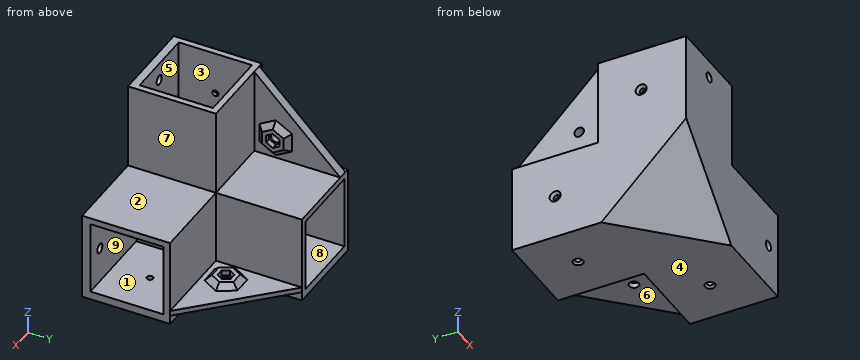
from build123d import *

# Parameters (mm, degrees)
ESQUISSE1_W                                       = 121.6
ESQUISSE1_H                                       = 121.6
BOSS_EXTRU_1_DEPTH                                = 60.8
ESQUISSE2_W                                       = 60.8
ESQUISSE2_H                                       = 60.8
ENL_V_MAT_EXTRU_1_DEPTH                           = 149.928976361
ESQUISSE3_W                                       = 60.8
ESQUISSE3_H                                       = 60.8
ENL_V_MAT_EXTRU_2_DEPTH                           = 106.3086891
ESQUISSE4_W                                       = 60.8
ESQUISSE4_H                                       = 60.8
ENL_V_MAT_EXTRU_3_DEPTH                           = 106.3086891
ESQUISSE5_W                                       = 51.8
ESQUISSE5_H                                       = 51.8
ENL_V_MAT_EXTRU_4_DEPTH                           = 60.8
ESQUISSE6_W                                       = 51.8
ESQUISSE6_H                                       = 51.8
ENL_V_MAT_EXTRU_5_DEPTH                           = 60.8
ESQUISSE7_W                                       = 51.8
ESQUISSE7_H                                       = 51.8
ENL_V_MAT_EXTRU_6_DEPTH                           = 60.8
BOSS_EXTRU_8_DEPTH                                = 1.35
FRAISAGE_POUR_VIS_T_TE_FRAIS_E_BOMB_E_D           = 4.3053
FRAISAGE_POUR_VIS_T_TE_FRAIS_E_BOMB_E_DEPTH       = 20
FRAISAGE_POUR_VIS_T_TE_FRAIS_E_BOMB_E_CSINK_D     = 7.0866
FRAISAGE_POUR_VIS_T_TE_FRAIS_E_BOMB_E_CSINK_ANGLE = 82
FRAISAGE_POUR_VIS_T_TE_FRAIS_E_BOMB_E_TIP         = 1.293442612
FRAISAGE_POUR_VIS_T_TE_FRAIS_E_6_PAN_D            = 4.3053
FRAISAGE_POUR_VIS_T_TE_FRAIS_E_6_PAN_DEPTH        = 20
FRAISAGE_POUR_VIS_T_TE_FRAIS_E_6_PAN_CSINK_D      = 7.7978
FRAISAGE_POUR_VIS_T_TE_FRAIS_E_6_PAN_CSINK_ANGLE  = 82
FRAISAGE_POUR_VIS_T_TE_FRAIS_E_6_PAN_TIP          = 1.293442612
BOSS_EXTRU_3_DEPTH                                = 10
ENL_V_MAT_EXTRU_13_DEPTH                          = 6.35
BOSS_EXTRU_2_DEPTH                                = 10
ENL_V_MAT_EXTRU_12_DEPTH                          = 3.3
D_GAGEMENT_1_42_D                                 = 6.7564
D_GAGEMENT_1_42_DEPTH                             = 20
D_GAGEMENT_1_42_TIP                               = 2.029827343
D_GAGEMENT_1_43_D                                 = 6.7564
D_GAGEMENT_1_43_DEPTH                             = 20
D_GAGEMENT_1_43_TIP                               = 2.029827343
BOSS_EXTRU_5_DEPTH                                = 4
CHANFREIN3_SIZE                                   = 4
BOSS_EXTRU_6_DEPTH                                = 4
CHANFREIN4_SIZE                                   = 4
BOSS_EXTRU_7_DEPTH                                = 1.35
D_GAGEMENT_1_44_D                                 = 6.7564
D_GAGEMENT_1_44_DEPTH                             = 20
D_GAGEMENT_1_44_TIP                               = 2.029827343
CHANFREIN1_START                                  = -108
CHANFREIN1_OUTLINE_W                              = 77
CHANFREIN1_OUTLINE_H                              = 88
CHANFREIN1_DEPTH                                  = 35.773481324


with BuildPart() as part:
    # Esquisse1 → Boss.-Extru.1 (new, symmetric)
    with BuildSketch(Plane.XY):
        Rectangle(ESQUISSE1_W, ESQUISSE1_H)
    extrude(amount=BOSS_EXTRU_1_DEPTH, both=True)

    # Esquisse2 → Enlèv. mat.-Extru.1 (cut, through all)
    with BuildSketch(Plane.XY.offset(60.8)):
        with Locations((30.4, 30.4)):
            Rectangle(ESQUISSE2_W, ESQUISSE2_H)
    extrude(amount=-ENL_V_MAT_EXTRU_1_DEPTH, mode=Mode.SUBTRACT)

    # Esquisse3 → Enlèv. mat.-Extru.2 (cut, through all)
    with BuildSketch(Plane(origin=(0, 0, 0), x_dir=(0, 0, -1), z_dir=(1, 0, 0))):
        with Locations((-30.4, 30.4)):
            Rectangle(ESQUISSE3_W, ESQUISSE3_H)
    extrude(amount=-ENL_V_MAT_EXTRU_2_DEPTH, mode=Mode.SUBTRACT)

    # Esquisse4 → Enlèv. mat.-Extru.3 (cut, through all)
    with BuildSketch(Plane(origin=(0, 0, 0), x_dir=(1, 0, 0), z_dir=(0, 1, 0))):
        with Locations((30.4, -30.4)):
            Rectangle(ESQUISSE4_W, ESQUISSE4_H)
    extrude(amount=-ENL_V_MAT_EXTRU_3_DEPTH, mode=Mode.SUBTRACT)

    # Esquisse5 → Enlèv. mat.-Extru.4 (cut)
    with BuildSketch(Plane.XY.offset(60.8)):
        with Locations((-30.4, -30.4)):
            Rectangle(ESQUISSE5_W, ESQUISSE5_H)
    extrude(amount=-ENL_V_MAT_EXTRU_4_DEPTH, mode=Mode.SUBTRACT)

    # Esquisse6 → Enlèv. mat.-Extru.5 (cut)
    with BuildSketch(Plane(origin=(60.8, 0, 0), x_dir=(0, 0, -1), z_dir=(1, 0, 0))):
        with Locations((30.4, -30.4)):
            Rectangle(ESQUISSE6_W, ESQUISSE6_H)
    extrude(amount=-ENL_V_MAT_EXTRU_5_DEPTH, mode=Mode.SUBTRACT)

    # Esquisse7 → Enlèv. mat.-Extru.6 (cut)
    with BuildSketch(Plane(origin=(0, 60.8, 0), x_dir=(1, 0, 0), z_dir=(0, 1, 0))):
        with Locations((-30.4, 30.4)):
            Rectangle(ESQUISSE7_W, ESQUISSE7_H)
    extrude(amount=-ENL_V_MAT_EXTRU_6_DEPTH, mode=Mode.SUBTRACT)

    # Esquisse40 → Boss.-Extru.8 (add)
    with BuildSketch(Plane(origin=(0, 0, -60.8), x_dir=(-1, 0, 0), z_dir=(0, 0, -1))):
        Polygon((0, 0), (-60.8, 0), (-60.8, -60.8), (60.8, -60.8), (60.8, 60.8), (0, 60.8), align=None)
    extrude(amount=BOSS_EXTRU_8_DEPTH)

    # Fraisage pour vis à tête fraisée bombée #61
    with Locations(Plane(origin=(0, 0, -62.15), x_dir=(-1, 0, 0), z_dir=(0, 0, -1))):
        with Locations((-30.4, -30.4), (30.4, 30.4)):
            CounterSinkHole(FRAISAGE_POUR_VIS_T_TE_FRAIS_E_BOMB_E_D / 2, FRAISAGE_POUR_VIS_T_TE_FRAIS_E_BOMB_E_CSINK_D / 2, depth=FRAISAGE_POUR_VIS_T_TE_FRAIS_E_BOMB_E_DEPTH, counter_sink_angle=FRAISAGE_POUR_VIS_T_TE_FRAIS_E_BOMB_E_CSINK_ANGLE)
            with Locations((0, 0, -(FRAISAGE_POUR_VIS_T_TE_FRAIS_E_BOMB_E_DEPTH + FRAISAGE_POUR_VIS_T_TE_FRAIS_E_BOMB_E_TIP / 2))):  # 118° drill point
                Cone(0, FRAISAGE_POUR_VIS_T_TE_FRAIS_E_BOMB_E_D / 2, FRAISAGE_POUR_VIS_T_TE_FRAIS_E_BOMB_E_TIP, mode=Mode.SUBTRACT)

    # Fraisage pour vis à tête fraisée à 6 pans creux #61
    with Locations(Plane.ZY.offset(60.8)):
        with Locations((30.4, -30.4), (-31.075, 30.4)):
            CounterSinkHole(FRAISAGE_POUR_VIS_T_TE_FRAIS_E_6_PAN_D / 2, FRAISAGE_POUR_VIS_T_TE_FRAIS_E_6_PAN_CSINK_D / 2, depth=FRAISAGE_POUR_VIS_T_TE_FRAIS_E_6_PAN_DEPTH, counter_sink_angle=FRAISAGE_POUR_VIS_T_TE_FRAIS_E_6_PAN_CSINK_ANGLE)
            with Locations((0, 0, -(FRAISAGE_POUR_VIS_T_TE_FRAIS_E_6_PAN_DEPTH + FRAISAGE_POUR_VIS_T_TE_FRAIS_E_6_PAN_TIP / 2))):  # 118° drill point
                Cone(0, FRAISAGE_POUR_VIS_T_TE_FRAIS_E_6_PAN_D / 2, FRAISAGE_POUR_VIS_T_TE_FRAIS_E_6_PAN_TIP, mode=Mode.SUBTRACT)

    # Esquisse21 → Boss.-Extru.3 (add)
    with BuildSketch(Plane(origin=(0, 0, -62.15), x_dir=(-1, 0, 0), z_dir=(0, 0, -1))):
        Polygon((0, 0), (-60.8, 0), (0, 60.8), align=None)
    extrude(amount=-BOSS_EXTRU_3_DEPTH)

    # Esquisse31 → Enlèv. mat.-Extru.13 (cut)
    with BuildSketch(Plane(origin=(0, 0, -62.15), x_dir=(-1, 0, 0), z_dir=(0, 0, -1))):
        Polygon((0, 60.8), (0, 0), (-60.8, 0), align=None)
    extrude(amount=-ENL_V_MAT_EXTRU_13_DEPTH, mode=Mode.SUBTRACT)

    # Esquisse17 → Boss.-Extru.2 (add)
    with BuildSketch(Plane.ZY.offset(60.8)):
        Polygon((0, 0), (60.8, 0), (0, 60.8), align=None)
    extrude(amount=-BOSS_EXTRU_2_DEPTH)

    # Esquisse26 → Enlèv. mat.-Extru.12 (cut)
    with BuildSketch(Plane.ZY.offset(60.8)):
        Polygon((0, 60.8), (0, 0), (60.8, 0), align=None)
    extrude(amount=-ENL_V_MAT_EXTRU_12_DEPTH, mode=Mode.SUBTRACT)

    # Dégagement 1/42
    with Locations(Plane.ZY.offset(57.5)):
        with Locations((15.2, 15.2)):
            Hole(D_GAGEMENT_1_42_D / 2, depth=D_GAGEMENT_1_42_DEPTH)
            with Locations((0, 0, -(D_GAGEMENT_1_42_DEPTH + D_GAGEMENT_1_42_TIP / 2))):  # 118° drill point
                Cone(0, D_GAGEMENT_1_42_D / 2, D_GAGEMENT_1_42_TIP, mode=Mode.SUBTRACT)

    # Dégagement 1/43
    with Locations(Plane(origin=(0, 0, -55.8), x_dir=(-1, 0, 0), z_dir=(0, 0, -1))):
        with Locations((-15.2, 15.2)):
            Hole(D_GAGEMENT_1_43_D / 2, depth=D_GAGEMENT_1_43_DEPTH)
            with Locations((0, 0, -(D_GAGEMENT_1_43_DEPTH + D_GAGEMENT_1_43_TIP / 2))):  # 118° drill point
                Cone(0, D_GAGEMENT_1_43_D / 2, D_GAGEMENT_1_43_TIP, mode=Mode.SUBTRACT)

    # Esquisse30 → Boss.-Extru.5 (add)
    with BuildSketch(Plane(origin=(-50.8, 0, 0), x_dir=(0, 0, -1), z_dir=(1, 0, 0))):
        Polygon((-6.395408395, 15.2), (-10.797704197, 22.825), (-19.602295803, 22.825), (-24.004591605, 15.2), (-19.602295803, 7.575), (-10.797704197, 7.575), align=None)
        Polygon((-9.85951001, 15.2), (-12.529755005, 19.825), (-17.870244995, 19.825), (-20.54048999, 15.2), (-17.870244995, 10.575), (-12.529755005, 10.575), align=None, mode=Mode.SUBTRACT)
    extrude(amount=BOSS_EXTRU_5_DEPTH)

    # Chanfrein3
    chanfrein3_edges = [part.edges().sort_by_distance(p)[0] for p in [
        (-50.8, 7.575, 15.2),
        (-50.8, 11.3875, 8.596556296),
        (-50.8, 19.0125, 8.596556296),
        (-50.8, 22.825, 15.2),
        (-50.8, 11.3875, 21.803443704),
        (-50.8, 19.0125, 21.803443704),
    ]]
    chamfer(chanfrein3_edges, length=CHANFREIN3_SIZE - 0.0001)  # a hair under: the kernel refuses the full size

    # Esquisse36 → Boss.-Extru.6 (add)
    with BuildSketch(Plane.XY.offset(-52.15)):
        Polygon((19.602295803, 22.825), (10.797704197, 22.825), (6.395408395, 15.2), (10.797704197, 7.575), (19.602295803, 7.575), (24.004591605, 15.2), align=None)
        Polygon((20.54048999, 15.2), (17.870244995, 19.825), (12.529755005, 19.825), (9.85951001, 15.2), (12.529755005, 10.575), (17.870244995, 10.575), align=None, mode=Mode.SUBTRACT)
    extrude(amount=BOSS_EXTRU_6_DEPTH)

    # Chanfrein4
    chanfrein4_edges = [part.edges().sort_by_distance(p)[0] for p in [
        (8.596556296, 11.3875, -52.15),
        (8.596556296, 19.0125, -52.15),
        (15.2, 7.575, -52.15),
        (21.803443704, 11.3875, -52.15),
        (21.803443704, 19.0125, -52.15),
        (15.2, 22.825, -52.15),
    ]]
    chamfer(chanfrein4_edges, length=CHANFREIN4_SIZE - 0.0001)  # a hair under: the kernel refuses the full size

    # Esquisse39 → Boss.-Extru.7 (add)
    with BuildSketch(Plane.XZ.offset(60.8)):
        Polygon((0, 0), (0, 60.8), (-60.8, 60.8), (-60.8, -62.15), (60.8, -62.15), (60.8, 0), align=None)
    extrude(amount=BOSS_EXTRU_7_DEPTH)

    # Dégagement 1/44
    with Locations(Plane(origin=(0, -62.15, 0), x_dir=(-1, 0, 0), z_dir=(0, -1, 0))):
        with Locations((-48.3, 31.075), (30.4, -48.3)):
            Hole(D_GAGEMENT_1_44_D / 2, depth=D_GAGEMENT_1_44_DEPTH)
            with Locations((0, 0, -(D_GAGEMENT_1_44_DEPTH + D_GAGEMENT_1_44_TIP / 2))):  # 118° drill point
                Cone(0, D_GAGEMENT_1_44_D / 2, D_GAGEMENT_1_44_TIP, mode=Mode.SUBTRACT)

    # Chanfrein1: read off the stored shape, not the designer's step
    # Chanfrein1 outline → Chanfrein1 (cut)
    with BuildSketch(Plane(origin=(0, 0, 0), x_dir=(0.816496580927726, -0.40824829046386324, -0.40824829046386263), z_dir=(0.5773502691896256, 0.5773502691896264, 0.5773502691896255)).offset(CHANFREIN1_START)):
        with Locations((13.5, 0)):
            Rectangle(CHANFREIN1_OUTLINE_W, CHANFREIN1_OUTLINE_H)
    extrude(amount=CHANFREIN1_DEPTH, mode=Mode.SUBTRACT)


solid = part.part
Work out the finished part from the listing and answer in its coordinate system (mm). Face numbers are marked on the shaded views. A direction names the side the tool comes from. Round coordinates to 2 decimals unless told otherwise and drop trailing zeros. Order: outer loops, then holes, each group sorted by start corner. A loop starts at its lowest first (then second) coordinate and runs counter-clockwise, first axis right, second up. Notation, with made-up numbers: M 64.25,-25.75 L 116.25,-25.75 A15 cw 116.25,-16.75 Z; hole C 24,-10 d7. An arc over 180 degrees is marked long. One line per item, written item: value.
Q1. Find section D-D on x = -30.4. Write down the section's boundary in (y, z), then the cut area to 3 significant figures.
Derived:
outline: M -62.15,-32.55 L -32.55,-62.15 L 26.86,-62.15 L 28.25,-60.55 L 28.25,-56.3 L 0,-56.3 L 0,-4.5 L 60.8,-4.5 L 60.8,0 L 0,0 L 0,60.8 L -4.5,60.8 L -4.5,0 L -56.3,0 L -56.3,44.92 L -62.15,44.92 Z; M -62.15,51.68 L -56.3,51.68 L -56.3,60.8 L -62.15,60.8 Z; M 32.55,-60.55 L 33.94,-62.15 L 60.8,-62.15 L 60.8,-56.3 L 32.55,-56.3 Z
area: 4,620 mm²
Q2. Flat-ended cylindrical pins translate along their axes: pin 1 (1.9 mm diameter, centred on y = 35.5, z = -58, fed in from +X); pin 2 (12 mm diameter, centred on y = 34.5, z = 7.5, fed in from -X); pin 3 (4 mm diameter, centred on x = -30.4, z = 48.3, fed in from -Y); pin 4 (11 mm diameter, centred on x = 48.3, z = -31.075, fed in from -Y). Find the tip coordinate at first contact, or state that the pin passes through.
Derived:
pin 1: x = 0
pin 2: x = -57.5
pin 3: y = -4.5
pin 4: y = -62.15
Q3. Find section B-B on y = 42.5. Write down the section's boundary in (x, z).
Derived:
outline: M -60.8,-62.15 L 0,-62.15 L 0,-55.8 L 18.3,-55.8 L 18.3,-52.15 L 0,-52.15 L 0,0 L -50.8,0 L -50.8,18.3 L -57.5,18.3 L -57.5,0 L -60.8,0 Z; hole M -56.3,-56.3 L -4.5,-56.3 L -4.5,-4.5 L -56.3,-4.5 Z
Q4. Find section A-A on x = 15.2. Give the number of separate pieces and of enclosed holes in the cut face, then the cut area to 3 significant figures.
Derived:
separate pieces: 2
enclosed holes: 1
area: 1,360 mm²
Q5. Determine the mould class of the marked faces 1, 2, 3 and 4 for opening direction Z: released by +Z, released by -Z, zero draft, split by the parting line, or undercut.
Derived:
face 1: undercut
face 2: released by +Z
face 3: zero draft
face 4: released by -Z
Q6. For the marked faces 5, 6, 7, 8 and 9, determine the directions among +Z, -Z, +X, -X, +Y, -Y from which every point of the face is accessible in a straight line to the end or side of a thin tool.
Derived:
face 5: +Z
face 6: -Z, +X, +Y
face 7: +Z, +X, +Y, -Y
face 8: +Y
face 9: +X
Q7. Straight lines are drawn through the part: line 1 (Y direction, x = -25, z = 46); line 2 (X direction, y = -26.5, z = 14). For each, find the intervals that lie inside material, in ascending order.
Derived:
line 1: -62.15 to -56.3, -4.5 to 0
line 2: -60.8 to -56.3, -4.5 to 0
